Geometry: final body of the model. Coordinates: model frame, mm. A direction names the side the tool comes from. Give positions to 0.01 mm unless a question says otherwise; leave off trailing zeros. Write each loop counter-clockwise with the first axis right and the second up, starting at its lowest first coordinate (ties: lowest second). Pieces come first, ordered by that corner, then holes. Notation, with made-up numbers: M 84,-28.75 L 101,-28.75 A17 ccw 101,-12.75 Z; hole C -33,76.25 d7. An arc over 180 degrees is marked long. One line per question, with ' | ' between items.
from build123d import *

# Parameters (mm, degrees)
SKETCH1_W           = 2.92
SKETCH1_H           = 2.92
SKETCH1_R           = 2.52
SKETCH1_R_2         = 0.5
BOSS_EXTRUDE1_DEPTH = 3


with BuildPart() as part:
    # Sketch1 → Boss-Extrude1 (new body)
    with BuildSketch(Plane.XY):
        Polygon((13.5482559, 6.709731544), (8.5482559, 11.709731544), (-2.4517441, 11.709731544), (-7.4517441, 6.709731544), (-7.4517441, -7.790268456), (8.5482559, -7.790268456), (8.5482559, -10.790268456), (-7.4517441, -10.790268456), (-7.4517441, -13.790268456), (13.5482559, -13.790268456), align=None)
        with Locations((3.0482559, -3.330268456)):
            Rectangle(SKETCH1_W, SKETCH1_H, mode=Mode.SUBTRACT)
        with Locations((3.0482559, 2.709731544)):
            Circle(SKETCH1_R, mode=Mode.SUBTRACT)
        with Locations((3.0482559, 8.709731544)):
            Circle(SKETCH1_R_2, mode=Mode.SUBTRACT)
    extrude(amount=BOSS_EXTRUDE1_DEPTH)


solid = part.part
(1) Cut plane D-D, the plane y = -10.5. Return loops of the section in (x, z).
Working result:
outline: M 8.55,0 L 13.55,0 L 13.55,3 L 8.55,3 Z
(2) Cut plane B-B, the plane y = 1. Return loops of the section in (x, z), then the cut area to 3 significant figures.
Working result:
outline: M -7.45,0 L 1.2,0 L 1.2,3 L -7.45,3 Z; M 4.9,0 L 13.55,0 L 13.55,3 L 4.9,3 Z | area: 51.9 mm^2
(3) Draft query along Y for faces 4 (the face through (3, -1, 3)), 5 (the face through (3, -4.79, 1)), 6 (the face through (11.083, 9.175, 1.479)). Return one class per face: released by +Y, released by -Y, zero draft, split by the parting line, or undercut.
Working result:
face 4: zero draft | face 5: undercut | face 6: released by +Y
(4) Cut plane A-A, the plane x = -1.5. Return loops of the section in (y, z).
Working result:
outline: M -13.79,0 L -10.79,0 L -10.79,3 L -13.79,3 Z; M -7.79,0 L 11.71,0 L 11.71,3 L -7.79,3 Z
(5) Set-up query: faces 1 (the face through (1.588, -3, 1)), 2 (the face through (-4.92, 9.24, 1.48)), 3 (the face through (0, -7.79, 1)). Return all of +Z, -Z, +X, -X, +Y, -Y with unobstructed straight access to the full face (end or side cutting, diameter ignored); none if empty.
Working result:
face 1: +Z, -Z | face 2: +Z, -Z, -X, +Y | face 3: +Z, -Z, -X
(6) First-contact query: P1, Ø1.5, axis at y = -9.5, z = 1, coming from the -X side. Flat tip, straight axial feed; report the tip coordinate or a pass-through.
Working result:
P1: stops at x = 8.55
(7) Material intervals for L1, parallel to X at y = -4, z = 0.45; L2, parallel to Y at x = 7.25, z = 1.5; L3, parallel to Y at x = 4.75, z = 2.2, sorted ascending. Write a range as [from, to].
Working result:
L1: x = [-7.45, 1.59], [4.51, 13.55] | L2: y = [-13.79, -10.79], [-7.79, 11.71] | L3: y = [-13.79, -10.79], [-7.79, 0.85], [4.57, 11.71]
(8) Cut plane C-C, the plane z = 0.9. Return loops of the section in (x, y).
Working result:
outline: M -7.45,-13.79 L 13.55,-13.79 L 13.55,6.71 L 8.55,11.71 L -2.45,11.71 L -7.45,6.71 L -7.45,-7.79 L 8.55,-7.79 L 8.55,-10.79 L -7.45,-10.79 Z; hole C 3.05,2.71 d5.04; hole M 1.59,-4.79 L 4.51,-4.79 L 4.51,-1.87 L 1.59,-1.87 Z; hole C 3.05,8.71 d1
